CAD build for the part. Positions are in the model's coordinates, mm. A direction names the side the tool comes from. Round coordinates to 2 decimals unless told otherwise and drop trailing zeros. Write each loop counter-clockwise with the first axis right and the second up, starting at its lowest first coordinate (ties: lowest second). Pieces come first, ordered by that corner, then holes. Notation, with made-up numbers: (-9, -37) -> (6, -37) arc R21 ccw to (6, -30) -> close; hole circle Ø8 at (37, 4). An arc over 180 degrees is marked (long way). Put each result on its own line as item: value. Start each with the question number.
1. 3-axis set-ups, long thin cutter, end or side, ignore diameter. For faces 1 (the cylindrical face through (-18.83, 4.93, -27.4)), 2 (the flat face through (-17.4, 6, 3)), 3 (the cylindrical face through (22.253, 1.479, 25.121)): which of +Z, -Z, +X, -X, +Y, -Y reach the whole face in a straight line?
2. Saw through at C-C on y = 3.75. State how many separate pieces and enclosed holes the cut face has, and give its area (3 significant figures).
3. Flat gauge pins, fed straight in: P1, Ø10, axis at x = -24.5, z = 6.5, coming from the -Y side; P2, Ø0.8, axis at y = 6.5, z = 25.5, coming from the -X side; P3, Ø4.5, axis at x = 25, z = 25, coming from the -Y side; P4, Ø10, axis at x = 15, z = 9, coming from the +Y side. Where does each tip first touch, or does it go through?
4. Saw through at A-A on x = 1.5. List the corners of the cut face in (y, z).
5. Drill centre lines: line 1 (X direction, y = 7.75, z = -9.5); line 2 (X direction, y = 1, z = 6.5); line 3 (Z direction, x = 12, y = 1.75). Where is each one in solid material? Low to high. Write a range as from..to.
6. Saw through at B-B on z = -11. List the corners of the cut face in (x, y), and give its area (3 significant figures).
7. Saw through at D-D on z = -25. List the corners of the cut face in (x, y).
Autodesk Inventor part; units mm, degrees
ref_plane "Work Plane2" through (0, 5, 0) normal (0, 1, 0) x (1, 0, 0)
ref_plane "YZ Plane" through (0, 0, 0) normal (1, 0, 0) x (0, 1, 0)
ref_plane "XZ Plane" through (0, 0, 0) normal (0, 1, 0) x (-1, 0, 0)
sketch "Sketch1" plane through (0, 0, 0) normal (0, 1, 0) x (-1, 0, 0)
  line L0 (30, 30) -> (-30, 30)
  line L1 (-30, 30) -> (-30, -30)
  line L2 (-30, -30) -> (30, -30)
  line L3 (30, -30) -> (30, 30)
  line L4 (30, 30) -> (-30, -30) construction
  line L5 (-30, 30) -> (30, -30) construction
  point P0 (0, 0)
  dimension "d0" = 60
  dimension "d1" = 60
extrude "Extrusion1" add sketch "Sketch1" along normal blind 10
fillet "Fillet1" radius 7 4 edges at (30, 5, 30) (30, 5, -30) (-30, 5, 30) (-30, 5, -30)
sketch "Sketch2" plane through (0, 10, 0) normal (0, 1, 0) x (1, 0, 0)
  line L0 (-30, 30) -> (30, 30)
  line L1 (30, 30) -> (30, -30)
  line L2 (30, -30) -> (-30, -30)
  line L3 (-30, -30) -> (-30, 30)
  line L4 (-30, 30) -> (30, -30) construction
  line L5 (30, 30) -> (-30, -30) construction
  line L6 (25, -25) -> (25, 25)
  line L7 (25, 25) -> (-25, 25)
  line L8 (-25, 25) -> (-25, -25)
  line L9 (-25, -25) -> (25, -25)
  circle A0 centre (25, -25) radius 2.75
  circle A1 centre (-25, -25) radius 2.75
  circle A2 centre (25, 25) radius 2.75
  circle A3 centre (-25, 25) radius 2.75
  point P0 (0, 0)
  dimension "d5" = 5
  dimension "d6" = 5.5
  dimension "d7" = 5.5
  dimension "d8" = 5.5
  dimension "d9" = 5.5
extrude "Extrusion2" cut sketch "Sketch2" against normal blind 3 contours L9 A0 L6 | L6 A0 L9 | A2 L7 L6 | L6 L7 A2 | A1 L8 L9 | L9 L8 A1 | A3 L8 L7 | L7 L8 A3
sketch "Sketch7" plane through (0, 10, 0) normal (0, 1, 0) x (1, 0, 0)
  line L0 (-23, 30) -> (23, 30)
  line L1 (30, 23) -> (30, -23)
  line L2 (23, -30) -> (-23, -30)
  line L3 (-30, -23) -> (-30, 23)
  line L4 (-30, 30) -> (30, -30) construction
  line L5 (30, 30) -> (-30, -30) construction
  arc A0 (-23, 30) -> (-30, 23) centre (-23, 23) ccw
  arc A1 (-30, -23) -> (-23, -30) centre (-23, -23) ccw
  arc A2 (23, -30) -> (30, -23) centre (23, -23) ccw
  arc A3 (30, 23) -> (23, 30) centre (23, 23) ccw
  line L6 (23, 32) -> (-23, 32)
  arc A4 (-23, 32) -> (-32, 23) centre (-23, 23) ccw
  line L7 (-32, 23) -> (-32, -23)
  arc A5 (-32, -23) -> (-23, -32) centre (-23, -23) ccw
  line L8 (-23, -32) -> (23, -32)
  arc A6 (23, -32) -> (32, -23) centre (23, -23) ccw
  line L9 (32, -23) -> (32, 23)
  arc A7 (32, 23) -> (23, 32) centre (23, 23) ccw
  point P0 (0, 0)
  dimension "d47" = 7
  dimension "d48" = 2
extrude "Extrusion6" add sketch "Sketch7" against normal blind 10
sketch "Sketch11" plane through (0, 10, 0) normal (0, 1, 0) x (1, 0, 0)
  circle A0 centre (25, -25) radius 2.75
  line L0 (-25, 25) -> (25, 25)
  line L1 (25, 25) -> (25, -25)
  line L2 (25, -25) -> (-25, -25)
  line L3 (-25, -25) -> (-25, 25)
  line L4 (-25, 25) -> (25, -25) construction
  line L5 (25, 25) -> (-25, -25) construction
  line L6 (21, -21) -> (21, 16.2)
  line L7 (-19.4, -21) -> (21, -21)
  line L8 (-19.4, -21) -> (-19.4, 16.2)
  line L9 (21, 16.2) -> (-19.4, 16.2)
  line L10 (-17.4, 14.2) -> (-17.4, -19)
  line L11 (-17.4, -19) -> (19, -19)
  line L12 (19, -19) -> (19, 14.2)
  line L13 (19, 14.2) -> (-17.4, 14.2)
  point P0 (0, 0)
  dimension "d66" = 4
  dimension "d67" = 40.4
  dimension "d68" = 37.2
  dimension "d69" = 2
extrude "Extrusion9" cut sketch "Sketch11" against normal blind 2 contours L7 L8 L9 L6
sketch "Sketch12" plane through (0, 10, 0) normal (0, 1, 0) x (1, 0, 0)
  line L0 (-17.4, 14.2) -> (19, 14.2)
  line L1 (19, 14.2) -> (19, -19)
  line L2 (19, -19) -> (-17.4, -19)
  line L3 (-17.4, -19) -> (-17.4, 14.2)
  point P0 (0, 0)
extrude "Extrusion10" cut sketch "Sketch12" against normal blind 8
sketch "Sketch13" plane through (0, 10, 0) normal (0, 1, 0) x (1, 0, 0)
  line L0 (23, 32) -> (-23, 32)
  line L1 (-19.4, 18.2) -> (-19.4, 28)
  line L2 (-19.4, 28) -> (19, 28)
  line L3 (-19.4, 18.2) -> (19, 18.2)
  line L4 (32, -23) -> (32, 23)
  line L5 (21, 16.2) -> (21, -21)
  line L6 (28, 16.2) -> (23, 16.2)
  line L7 (23, 16.2) -> (23, -19)
  line L8 (28, -19) -> (28, 16.2)
  line L9 (23, -19) -> (28, -19)
  line L10 (21, -21) -> (-19.4, -21)
  line L11 (-23, -32) -> (23, -32)
  line L12 (19, -28) -> (19, -23)
  line L13 (19, -28) -> (-19.4, -28)
  line L14 (-19.4, -28) -> (-19.4, -23)
  line L15 (-19.4, -23) -> (19, -23)
  line L16 (19, 18.2) -> (19, 28)
  line L17 (19, 14.2) -> (19, -19)
  line L18 (-32, 23) -> (-32, -23)
  line L19 (-19.4, -21) -> (-19.4, 16.2)
  line L20 (-28, -19) -> (-28, 19.5)
  line L21 (-28, -19) -> (-21.4, -19)
  line L22 (-21.4, -19) -> (-21.4, 19.5)
  line L23 (-28, 19.5) -> (-21.4, 19.5)
  dimension "d77" = 2
  dimension "d78" = 4
  dimension "d81" = 2
  dimension "d84" = 2
  dimension "d87" = 4
  dimension "d88" = 4
  dimension "d89" = 2
  dimension "d90" = 38.5
extrude "Extrusion11" cut sketch "Sketch13" against normal through all
fillet "Fillet3" radius 2 16 edges at (-19.4, 5, -28) (-28, 5, -19.5) (23, 5, -16.2) (-19.4, 5, 23) (19, 5, -28) (-21.4, 5, -19.5) (28, 5, -16.2) (19, 5, 23) (19, 5, -18.2) (28, 5, 19) (19, 5, 28) (-21.4, 5, 19) (-19.4, 5, -18.2) (23, 5, 19) (-19.4, 5, 28) (-28, 5, 19)
fillet "Fillet3" radius 1 4 edges at (0.8, 2, -14.2) (19, 2, 2.4) (-17.4, 2, 2.4) (0.8, 2, 19)
ref_plane "Work Plane2" through (0, 5, 0) normal (0, 1, 0) x (1, 0, 0)
mirror "Mirror2" about plane through (0, 5, 0) normal (0, 1, 0) of "Extrusion2"
properties part number "20 pin IC holder2"
Return value:
1. face 1: +Y, -Y
1. face 2: +Y
1. face 3: -Y
2. separate pieces: 1
2. enclosed holes: 5
2. area: 1,830 mm^2
3. P1: stops at y = 0
3. P2: stops at x = -31.75
3. P3: stops at y = 3
3. P4: stops at y = 8
4. outline: (0, -32) -> (10, -32) -> (10, -28) -> (0, -28) -> close; (0, -18.2) -> (10, -18.2) -> (10, -16.2) -> (8, -16.2) -> (8, -14.2) -> (3, -14.2) arc R1 cw to (2, -13.2) -> (2, 18) arc R1 cw to (3, 19) -> (8, 19) -> (8, 21) -> (10, 21) -> (10, 23) -> (0, 23) -> close; (0, 28) -> (10, 28) -> (10, 32) -> (0, 32) -> close
5. line 1: x = -32..-28, -21.4..-17.4, 19..23, 28..32
5. line 2: x = -32..-28, -21.4..23, 28..32
5. line 3: z = -32..-28, -18.2..23, 28..32
6. outline: (-32, 0) -> (-28, 0) -> (-28, 10) -> (-32, 10) -> close; (-21.4, 0) -> (23, 0) -> (23, 10) -> (21, 10) -> (21, 8) -> (19, 8) -> (19, 3) arc R1 cw to (18, 2) -> (-16.4, 2) arc R1 cw to (-17.4, 3) -> (-17.4, 8) -> (-19.4, 8) -> (-19.4, 10) -> (-21.4, 10) -> close; (28, 0) -> (32, 0) -> (32, 10) -> (28, 10) -> close
6. area: 225 mm^2
7. outline: (-31.77, 0) -> (-27.75, 0) -> (-27.75, 3) -> (-22.25, 3) -> (-22.25, 0) -> (-19.4, 0) -> (-19.4, 10) -> (-22.25, 10) -> (-22.25, 7) -> (-27.75, 7) -> (-27.75, 10) -> (-31.77, 10) -> close; (19, 0) -> (22.25, 0) -> (22.25, 3) -> (27.75, 3) -> (27.75, 0) -> (31.77, 0) -> (31.77, 10) -> (27.75, 10) -> (27.75, 7) -> (22.25, 7) -> (22.25, 10) -> (19, 10) -> close
